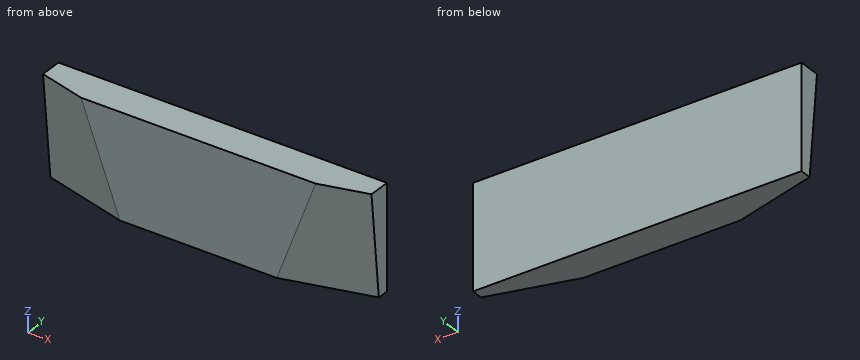
```python
from build123d import *

# Parameters (mm, degrees)
F0_W     = 482.6
F0_H     = 50.8
F1_DEPTH = 152.4


# Not quite as in the source:
# - a pattern or mirror of a feature is missing from the dataset's text; its kind, count and spacing are read off the source's solid


with BuildPart() as f1:
    # F0 (on Top) → F1 (new body)
    with BuildSketch(Plane.XY):
        Rectangle(F0_W, F0_H)
    extrude(amount=F1_DEPTH)

    # F4: sweep along a path in F3
    with BuildLine(Plane(origin=(-241.3, 0, 0), x_dir=(0, -1, 0), z_dir=(-1, 0, 0))) as f4_path:
        Line((15.9376427472, 242.2395817821), (-8.382, 0))
    # F2 (on face) → F4 (sweep, cut)
    with BuildSketch(Plane(origin=(0, 0, 0), x_dir=(1, 0, 0), z_dir=(0, 0, -1))):
        Polygon((-241.3, 25.4), (-241.3, -8.382), (-115.2238596187, 25.4), align=None)
    f4 = sweep(path=f4_path.line, mode=Mode.SUBTRACT)

    # F4_copies: F4 across plane
    add(f4.mirror(Plane(origin=(0, 0, 0), x_dir=(0, 0, 1), z_dir=(1, 0, 0))), mode=Mode.SUBTRACT)


solid = f1.part
```
Can you work these out from the model? Positions are in its coordinate system, mm. Round coordinates to 2 decimals unless told otherwise and drop trailing zeros. Loops run counter-clockwise (first coordinate to the right, second up) from the corner with the lowest first, then second, coordinate; pieces in that order, holes last.
Item 1: Suppose I cut it at A-A, the plane z = 101. Write out the boundary of the cut face in (x, y), then the cut area to 3 significant figures.
Item 2: Suppose I cut it at B-B, the plane x = 133.5. Write out the boundary of the cut face in (y, z).
Item 3: Suppose I cut it at D-D, the plane z = 36.5. Write out the boundary of the cut face in (x, y), then the cut area to 3 significant figures.
Item 4: Please list where these lines run through material, in increasing order: L1, parallel to Y at x = 166, z = 78; L2, parallel to Y at x = 192.5, z = 127.
Item 5: Suppose I cut it at C-C, the plane y = -21. Write out the boundary of the cut face in (x, z), then the cut area to 3 significant figures.
Item 6: Will this pin go through, and if not, where does the flat tip stop? pin 1 Ø4 at (y, z) = (-1.5, 87) entering from +X.
Reported:
1. outline: (-241.3, -1.76) - (-153.07, -25.4) - (153.07, -25.4) - (241.3, -1.76) - (241.3, 25.4) - (-241.3, 25.4) - close
1. area: 22,400 mm2
2. outline: (-25.4, 48.78) - (-20.5, 0) - (25.4, 0) - (25.4, 152.4) - (-25.4, 152.4) - close
3. outline: (-241.3, 4.72) - (-128.9, -25.4) - (128.9, -25.4) - (241.3, 4.72) - (241.3, 25.4) - (-241.3, 25.4) - close
3. area: 21,100 mm2
4. L1: y = -19.63 to 25.4
4. L2: y = -17.44 to 25.4
5. outline: (-188.75, 152.4) - (-131.64, 0) - (131.64, 0) - (188.75, 152.4) - close
5. area: 48,800 mm2
6. pin 1: stops at x = 241.3
